```python
from build123d import *

# Parameters (mm, degrees)
F0_W     = 6.14
F0_H     = 5
F1_DEPTH = 32
F2_W     = 6.14
F2_H     = 21.9306324124
F3_DEPTH = 5
F4_DEPTH = 7.4
F5_DEPTH = 7.4
F6_R     = 1.5


with BuildPart() as f1:
    # F0 (on Top) → F1 (new body)
    with BuildSketch(Plane.XY):
        Polygon((0, 15), (0, 0), (6, 0), (6, 10), (6, 15), align=None)
        with Locations((9.07, 12.5)):
            Rectangle(F0_W, F0_H)
        Polygon((12.14, 15), (12.14, 10), (12.14, 0), (17.14, 0), (17.14, 25), (58, 25), (58, 30), (17.14, 30), (17.14, 35), (52.157233721, 35), (52.957233721, 35), (54.8181005478, 35), (55.6181005478, 35), (58, 35), (58, 40), (12.14, 40), (12.14, 25), align=None)
        with BuildLine():
            ThreePointArc((54.8181005478, 35), (55.2181005478, 34.6), (55.6181005478, 35))
            Line((55.6181005478, 35), (54.8181005478, 35))
        make_face()
        with BuildLine():
            ThreePointArc((52.157233721, 35), (52.557233721, 34.6), (52.957233721, 35))
            Line((52.957233721, 35), (52.157233721, 35))
        make_face()
    extrude(amount=F1_DEPTH)

    # F2 (on face) → F3 (cut)
    with BuildSketch(Plane.XZ.offset(-10)):
        with Locations((9.07, 16.0346837938)):
            Rectangle(F2_W, F2_H)
    extrude(amount=-F3_DEPTH, mode=Mode.SUBTRACT)

    # F4 (add): a face of the model
    f4_faces = [f1.faces().sort_by_distance(p)[0] for p in [
        (37.57, 25, 16),
    ]]
    extrude(f4_faces, amount=F4_DEPTH)

    # F5 (cut): a face of the model
    f5_faces = [f1.faces().sort_by_distance(p)[0] for p in [
        (37.57, 30, 16),
    ]]
    extrude(f5_faces, amount=-F5_DEPTH, mode=Mode.SUBTRACT)

    # F6
    f6_edges = [f1.edges().sort_by_distance(p)[0] for p in [
        (12.14, 5, 32),
        (12.14, 27.5, 32),
        (12.14, 5, 0),
        (12.14, 27.5, 0),
        (0, 15, 16),
        (0, 0, 16),
        (0, 7.5, 0),
        (0, 7.5, 32),
        (17.14, 8.8, 0),
        (17.14, 28.8, 0),
        (17.14, 28.8, 32),
        (17.14, 8.8, 32),
        (37.57, 17.6, 32),
        (37.57, 17.6, 0),
        (35.07, 40, 0),
        (35.07, 40, 32),
        (58, 40, 16),
        (58, 17.6, 16),
    ]]
    fillet(f6_edges, radius=F6_R)


solid = f1.part
```
The listing builds one solid part. Answer for the finished solid, in the listing's coordinates (mm). A direction names the side the tool comes from. Round coordinates to 2 decimals unless told otherwise and drop trailing zeros. Write each loop counter-clockwise with the first axis right and the second up, starting at its lowest first coordinate (ties: lowest second). Pieces come first, ordered by that corner, then holes. Notation, with made-up numbers: (-2.75, 39.25) -> (15.25, 39.25) arc R13 ccw to (15.25, 45.25) -> close; hole circle Ø5 at (55.5, 48). An arc over 180 degrees is marked (long way). Write item = value, one per line.
1) For a pull along X with two mould halves and no side action, classify faces 1 (the cylindrical face through (57.57, 18.05, 16.22)), 2 (the cylindrical face through (0.45, 0.43, 16.22)), 3 (the flat face through (12.14, 20, 16)) as released by +X, released by -X, zero draft, split by the parting line, or undercut.
Check values:
face_1 = released by +X
face_2 = released by -X
face_3 = undercut
2) Given pin 1 (5 mm diameter, centred on y = 22.5, z = 9.5, fed in from -X); pin 2 (9.5 mm diameter, centred on x = 31, z = 15, fed in from -Y); pin 3 (9 mm diameter, centred on y = 7, z = 19, fed in from +X), each flat-ended and moving along its own axis, determine where each tip first touches the part or whether it passes through.
Check values:
pin_1 = 12.14
pin_2 = 17.6
pin_3 = 17.14
3) Straight lines are drawn through the part: line 1 along X through (y, z) = (3, 21); line 2 along Y through (x, z) = (26.5, 5.5); line 3 along X through (y, z) = (20.5, 22). For each, find the intervals that lie inside material, in ascending order. Write a range as [from, to].
Check values:
line_1 = [0, 6], [12.14, 17.14]
line_2 = [17.6, 22.6], [35, 40]
line_3 = [12.14, 58]
4) Which of the six approach directions +Z, -Z, +X, -X, +Y, -Y give full straight-line access (tool end or side, diameter ignored) to faces 4 (the flat face through (54, 35, 16)), 5 (the flat face through (6, 7, 16)), 6 (the cylindrical face through (16.71, 9.68, 0.45))?
Check values:
face_4 = +Z, -Z
face_5 = -Y
face_6 = -Z, +X, -Y
5) Section D-D on y = 25 is taken. Write down the section's boundary in (x, z), plus the area to 3 significant figures.
Check values:
outline = (12.14, 1.5) arc R1.5 ccw to (13.64, 0) -> (15.64, 0) arc R1.5 ccw to (17.14, 1.5) -> (17.14, 30.5) arc R1.5 ccw to (15.64, 32) -> (13.64, 32) arc R1.5 ccw to (12.14, 30.5) -> close
area = 158 mm²
6) Section B-B on y = 6 is taken. Write down the section's boundary in (x, z), plus the area to 3 significant figures.
Check values:
outline = (0, 1.5) arc R1.5 ccw to (1.5, 0) -> (6, 0) -> (6, 32) -> (1.5, 32) arc R1.5 ccw to (0, 30.5) -> close; (12.14, 1.5) arc R1.5 ccw to (13.64, 0) -> (15.64, 0) arc R1.5 ccw to (17.14, 1.5) -> (17.14, 30.5) arc R1.5 ccw to (15.64, 32) -> (13.64, 32) arc R1.5 ccw to (12.14, 30.5) -> close
area = 349 mm²
7) Section C-C on x = 23 is taken. Write down the section's boundary in (y, z), plus the area to 3 significant figures.
Check values:
outline = (17.6, 1.5) arc R1.5 ccw to (19.1, 0) -> (22.6, 0) -> (22.6, 32) -> (19.1, 32) arc R1.5 ccw to (17.6, 30.5) -> close; (35, 0) -> (38.5, 0) arc R1.5 ccw to (40, 1.5) -> (40, 30.5) arc R1.5 ccw to (38.5, 32) -> (35, 32) -> close
area = 318 mm²
8) Section A-A on z = 23 is taken. Write down the section's boundary in (x, y).
Check values:
outline = (0, 1.5) arc R1.5 ccw to (1.5, 0) -> (6, 0) -> (6, 15) -> (1.5, 15) arc R1.5 ccw to (0, 13.5) -> close; (12.14, 0) -> (17.14, 0) -> (17.14, 17.6) -> (56.5, 17.6) arc R1.5 ccw to (58, 19.1) -> (58, 22.6) -> (17.14, 22.6) -> (17.14, 35) -> (52.16, 35) arc R0.4 ccw to (52.96, 35) -> (54.82, 35) arc R0.4 ccw to (55.62, 35) -> (58, 35) -> (58, 38.5) arc R1.5 ccw to (56.5, 40) -> (12.14, 40) -> close
